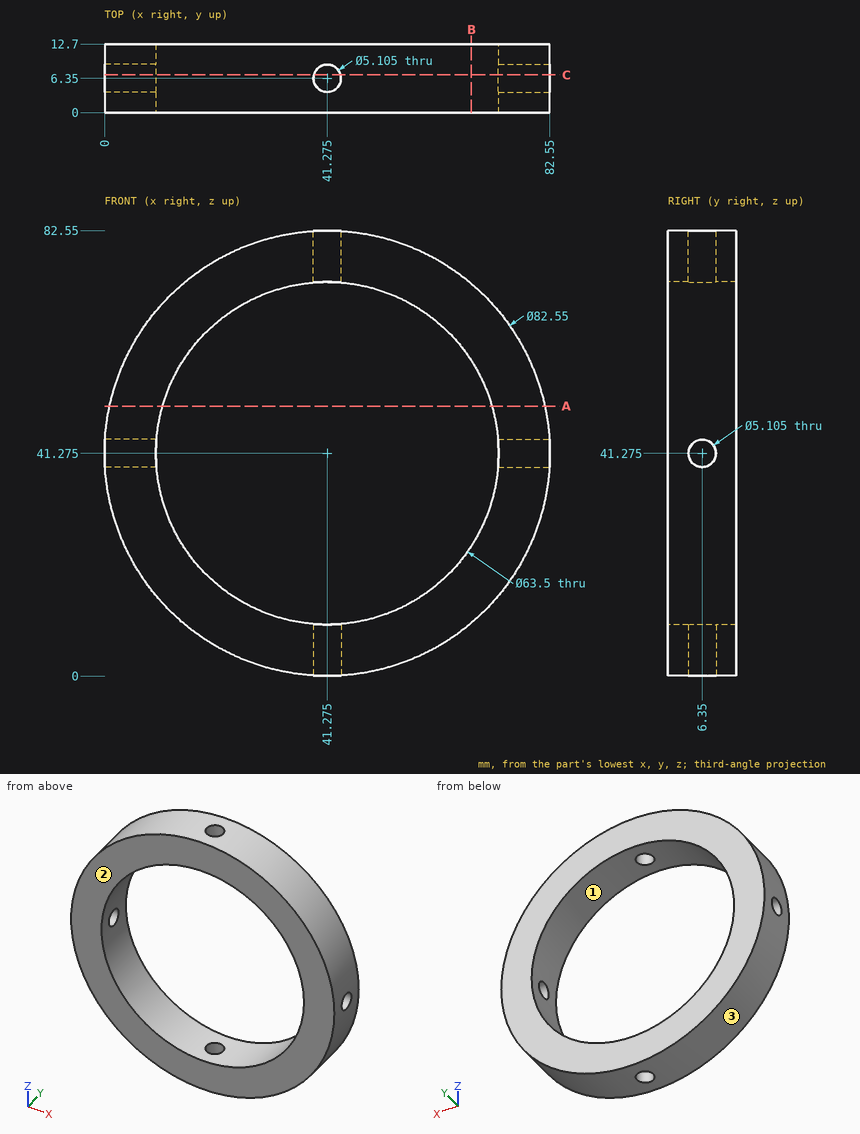
Print and shaded views of the part. All mm, measured from the part's lowest x, y and z. Round coordinates to 2 decimals unless told otherwise and drop trailing zeros. Write each loop counter-clockwise with the first axis right and the second up, starting at its lowest first coordinate (ties: lowest second). Pieces come first, ordered by that corner, then holes.
(1) Probe line 1 along Z through (x, y) = (34.5, 8.25); line 2 along X through (y, z) = (6.35, 4.5) (1 decimal); line 3 along X through (y, z) = (9.25, 29) (1 decimal). List the from-to ranges inside material, lowest first.
(2) Slice it at A-A, the plane z = 50. Write the cut outline in (x, y), and give its area (3 significant figures).
(3) Mould opens along Z. For the marked faces 1, 2 and 3 say: pulls with the +Z half, pulls with the -Z half, needs draft (parallel to the pull), parting line crosses it, or undercut.
(4) Drop flat-ended pins along their axis: P1, Ø3, axis at x = 41.275, y = 6.35, coming from the -Z side; P2, Ø5, axis at y = 3.5, z = 47, coming from the +X side; P3, Ø4, axis at x = 28, y = 4.5, coming from the -Z side; P4, Ø5, axis at x = 33.5, y = 2, coming from the -Z side. Give the stop position or say it passes through.
(5) Slice it at B-B, the plane x = 68. Write the cut outline in (y, z).
(6) Slice it at C-C, the plane y = 7. Count the separate pieces of the cut face and the enclosed holes in it, and give its area (3 significant figures).
From the geometry:
1. line 1: z = 0.56 to 10.26, 72.29 to 81.99
1. line 2: x = 22.5 to 38.7, 43.8 to 60
1. line 3: x = 1.9 to 12, 70.6 to 80.7
2. outline: (0.93, 0) - (10.75, 0) - (10.75, 12.7) - (0.93, 12.7) - close; (71.8, 0) - (81.62, 0) - (81.62, 12.7) - (71.8, 12.7) - close
2. area: 249 mm2
3. face 1: undercut
3. face 2: needs draft
3. face 3: parting line crosses it
4. P1: passes through
4. P2: stops at x = 82.42
4. P3: stops at z = 1.57
4. P4: stops at z = 0.34
5. outline: (0, 9.82) - (12.7, 9.82) - (12.7, 24.13) - (0, 24.13) - close; (0, 58.42) - (12.7, 58.42) - (12.7, 72.73) - (0, 72.73) - close
6. separate pieces: 4
6. enclosed holes: 0
6. area: 2,000 mm2
